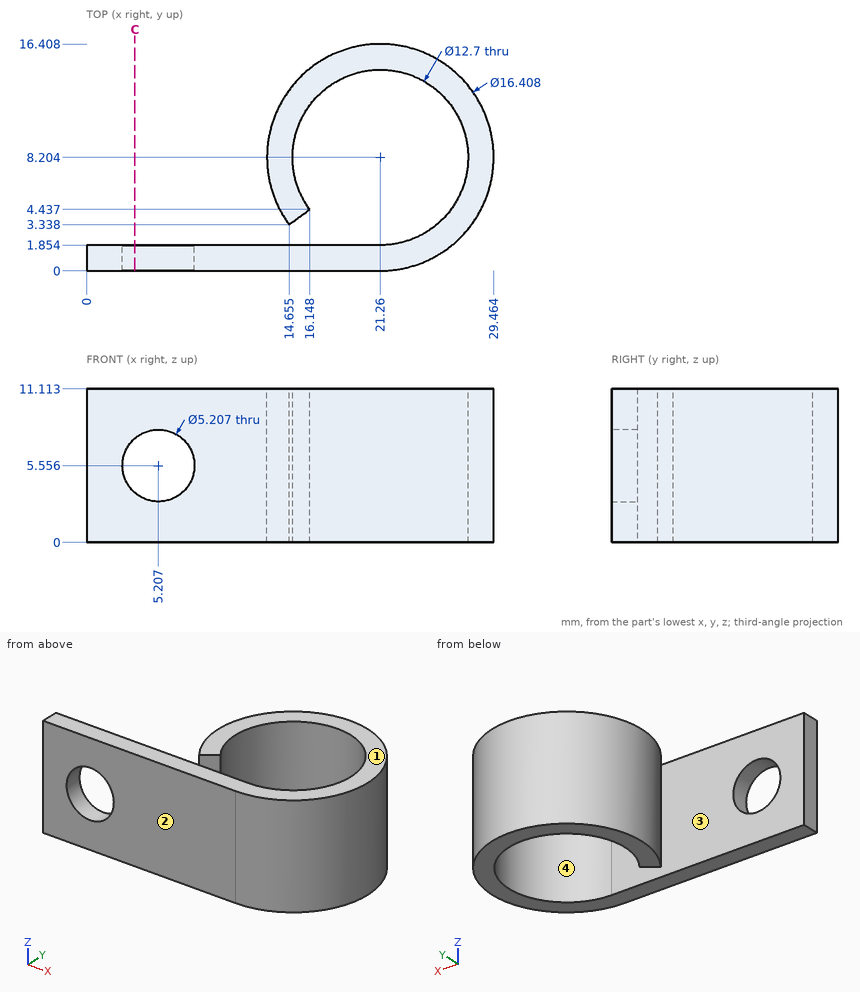
The drawing under review shows one solid part. Ordinate dimensions are in mm from its lowest x, y, z. Coordinates: 2 decimals unless noted, no trailing zeros. Write each loop counter-clockwise with the first axis right and the second up, starting at its lowest first coordinate (ties: lowest second). Pieces come first, ordered by that corner, then holes. Notation, with made-up numbers: (45.25, 81) - (71.25, 81) arc R26 ccw to (71.25, 119) - close; hole circle Ø4 at (-23.5, 47). An arc over 180 degrees is marked (long way). Put each result on its own line as item: value.
1. Mouldability with a two-part tool opening along Y and no side actions: class the marked faces 1, 2, 3 and 4 as released by +Y, released by -Y, zero draft, split by the parting line, or undercut.
Values found:
face 1: zero draft
face 2: released by -Y
face 3: undercut
face 4: undercut
2. Add section C-C, the plane x = 3.5. Give the boundary of the cut face in (y, z) (1 decimal), then the cut area to 3 significant figures.
Values found:
outline: (0, 0) - (1.9, 0) - (1.9, 3.6) - (0, 3.6) - close; (0, 7.5) - (1.9, 7.5) - (1.9, 11.1) - (0, 11.1) - close
area: 13.3 mm²
3. Wall thickness on probe 1 along X at (y, z) = (8, 8); probe 2 along X at (y, z) = (4, 4.5) (1 decimal); probe 3 along Y at (x, z) = (22.25, 4): over which ranges is each line inside the solid? List them lowest first.
Values found:
probe 1: 13.06 to 14.91, 27.61 to 29.46
probe 2: 14.2 to 15.6, 26 to 28.3
probe 3: 0.06 to 1.93, 14.48 to 16.35
4. For pin 1 (5.5 mm diameter, centred on x = 6.5, z = 4.5, fed in from +Y); pin 2 (2 mm diameter, centred on y = 7, z = 7, fed in from +X); pin 3 (1 mm diameter, centred on y = 5.5, z = 2, fed in from -X); pin 4 (6 mm diameter, centred on x = 16.5, y = 6.5, fed in from -Z), all flat-tipped, find the tip position at first contact; note any pin that passes through.
Values found:
pin 1: y = 1.85
pin 2: x = 29.46
pin 3: x = 13.36
pin 4: z = 0
